from build123d import *

# Parameters (mm, degrees)
SKETCH1_W                 = 19.05
SKETCH1_H                 = 19.05
SKETCH1_W_2               = 15.875
SKETCH1_H_2               = 15.875
TUBE_DEPTH                = 457.4032
SKETCH2_R                 = 2.8956
TOPPLATEHOLES_DEPTH       = 20.05
LPATTERN1_COUNT           = 4
LPATTERN1_PITCH           = 110.202133333
SKETCH3_R                 = 2.8956
SIDEPLATEHOLEMASTER_DEPTH = 20.05
LPATTERN2_COUNT           = 4
LPATTERN2_PITCH           = 127.067733333


with BuildPart() as part:
    # Sketch1 → Tube (new body)
    with BuildSketch(Plane(origin=(0, 0, 0), x_dir=(1, 0, 0), z_dir=(0, 1, 0))):
        Rectangle(SKETCH1_W, SKETCH1_H)
        Rectangle(SKETCH1_W_2, SKETCH1_H_2, mode=Mode.SUBTRACT)
    extrude(amount=TUBE_DEPTH)

    # Sketch2 → TopPlateHoles (cut, through all)
    with BuildSketch(Plane.XY.offset(9.525)):
        with Locations((0, 394.0048)):
            Circle(SKETCH2_R)
    topplateholes = extrude(amount=-TOPPLATEHOLES_DEPTH, mode=Mode.SUBTRACT)

    # LPattern1: TopPlateHoles ×4
    with Locations(*[(0, -i * LPATTERN1_PITCH, 0) for i in range(1, LPATTERN1_COUNT)]):
        add(topplateholes, mode=Mode.SUBTRACT)

    # Sketch3 → SidePlateHoleMaster (cut, through all)
    with BuildSketch(Plane.ZY.offset(9.525)):
        with Locations((0, 419.3032)):
            Circle(SKETCH3_R)
    sideplateholemaster = extrude(amount=-SIDEPLATEHOLEMASTER_DEPTH, mode=Mode.SUBTRACT)

    # LPattern2: SidePlateHoleMaster ×4
    with Locations(*[(0, -i * LPATTERN2_PITCH, 0) for i in range(1, LPATTERN2_COUNT)]):
        add(sideplateholemaster, mode=Mode.SUBTRACT)


solid = part.part
Check sheet for the modelled part. Datum: model origin and axes. Units: mm. A direction names the side the tool comes from. Round coordinates to 2 decimals unless told otherwise and drop trailing zeros. Loops run counter-clockwise (first coordinate to the right, second up) from the corner with the lowest first, then second, coordinate; pieces in that order, holes last. Notation, with made-up numbers: (49, 21.5) - (73, 21.5) arc R28 ccw to (73, 52.5) - close; hole circle Ø1 at (40.5, -8.5). An arc over 180 degrees is marked (long way). Answer as CSV lines item,"result". Start each with the question number.
Item 1: Release check for a two-part mould opening along Z. For faces 1 (the flat face through (9.525, 225, 0)), 2 (the flat face through (0, 225, -9.525)), 3 (the flat face through (7.938, 225, 0)), 4 (the flat face through (0, 225, 9.525)) record: +Z half, -Z half, draft (parallel to the pull), parting line (faces both ways), or undercut.
Item 2: Scan lines: line 1 (Y direction, x = 8.8, z = 0); line 2 (Y direction, x = 0, z = -8.8); line 3 (X direction, y = 109, z = -4) (1 decimal). Record each from-to range of solid material in increasing order. Write a range as [from, to].
Item 3: Section check A-A (y = 325.5). Record the boundary of the cut face in (x, z) (1 decimal), and give its area (3 significant figures).
Item 4: Section check B-B (x = 0). Count the separate pieces of the cut face and the enclosed holes in it, and give its area (3 significant figures).
Item 5: Set-up check for faces 5 (the flat face through (-7.938, 225, 0)), 6 (the flat face through (-9.525, 225, 0)): record each of +Z, -Z, +X, -X, +Y, -Y from which the full face is reachable in a straight line by a thin tool's end or side.
Item 6: Depth check by flat-ended pin: P1, Ø5, axis at x = 0, y = 283.8, coming from the -Z side. Enter the tip coordinate at first touch or a pass-through.
Report:
1,face 1,"draft"
1,face 2,"-Z half"
1,face 3,"undercut"
1,face 4,"+Z half"
2,line 1,"y = [0, 35.2], [41, 162.27], [168.06, 289.34], [295.13, 416.41], [422.2, 457.4]"
2,line 2,"y = [0, 60.5], [66.29, 170.7], [176.5, 280.91], [286.7, 391.11], [396.9, 457.4]"
2,line 3,"x = [-9.5, -7.9], [7.9, 9.5]"
3,outline,"(-9.5, -9.5) - (9.5, -9.5) - (9.5, 9.5) - (-9.5, 9.5) - close; hole (-7.9, -7.9) - (7.9, -7.9) - (7.9, 7.9) - (-7.9, 7.9) - close"
3,area,"111 mm2"
4,separate pieces,"10"
4,enclosed holes,"0"
4,area,"1,380 mm2"
5,face 5,"+Y, -Y"
5,face 6,"+Z, -Z, -X, +Y, -Y"
6,P1,"passes through"
